Could you check a few things on this model? Use its own coordinates, in mm. A direction names the side the tool comes from. Coordinates: 2 decimals unless noted, no trailing zeros. Loops run counter-clockwise (first coordinate to the right, second up) from the corner with the lowest first, then second, coordinate; pieces in that order, holes last. Notation, with made-up numbers: M -16.5,-12 L 32.5,-12 A15 cw 32.5,13 Z; hole C 70.25,81 d6. An arc over 180 degrees is marked long. Return JSON: item names as keys, results as strings. Group by question number.
from build123d import *

# Parameters (mm, degrees)
SKETCH1_R                      = 27.4955
SKETCH1_R_2                    = 2
SKETCH1_R_3                    = 52.3875
SKETCH1_R_4                    = 3.3
BOSS_EXTRUDE1_DEPTH            = 9.525
M8_CLEARANCE_HOLE1_D           = 9
M8_CLEARANCE_HOLE1_CSINK_D     = 9.05
M8_CLEARANCE_HOLE1_CSINK_ANGLE = 90
CIRPATTERN1_COUNT              = 9


with BuildPart() as part:
    # Sketch1 → Boss-Extrude1 (new body)
    with BuildSketch(Plane(origin=(0, 0, 0), x_dir=(-1, 0, 0), z_dir=(0, 1, 0))):
        with BuildLine():
            Line((-663.918846707, 4.476573271), (-466.57213203, 18.457038772))
            ThreePointArc((-466.57213203, 18.457038772), (-462.140898161, 18.198594818), (-457.960546806, 16.706184206))
            ThreePointArc((-457.960546806, 16.706184206), (-450.250504554, 16.184701691), (-444.691176426, 21.552249203))
            Line((-444.691176426, 21.552249203), (-395.545795992, 142.743123059))
            ThreePointArc((-395.545795992, 142.743123059), (-394.045633102, 172.997422567), (-411.692336104, 197.617881552))
            ThreePointArc((-411.692336104, 197.617881552), (-413.372500119, 198.071242365), (-414.950136715, 197.336701751))
            Line((-414.950136715, 197.336701751), (-420.215020333, 192.071818133))
            ThreePointArc((-420.215020333, 192.071818133), (-427.298656721, 190.662795249), (-431.31121441, 196.668012211))
            Line((-431.31121441, 196.668012211), (-431.31121441, 203.240745001))
            ThreePointArc((-431.31121441, 203.240745001), (-431.968379704, 204.945600851), (-433.59982344, 205.768273949))
            ThreePointArc((-433.59982344, 205.768273949), (-438.15, 205.994), (-442.70017656, 205.768273949))
            ThreePointArc((-442.70017656, 205.768273949), (-444.331620296, 204.945600851), (-444.98878559, 203.240745001))
            Line((-444.98878559, 203.240745001), (-444.98878559, 196.668012211))
            ThreePointArc((-444.98878559, 196.668012211), (-451.48878559, 190.168012211), (-457.98878559, 196.668012211))
            Line((-457.98878559, 196.668012211), (-457.98878559, 197.245022653))
            ThreePointArc((-457.98878559, 197.245022653), (-459.278285753, 199.455870942), (-461.837486501, 199.421924563))
            ThreePointArc((-461.837486501, 199.421924563), (-464.019895008, 198.024699819), (-466.120112298, 196.506730383))
            Line((-466.120112298, 196.506730383), (-526.629683433, 150.121113421))
            ThreePointArc((-526.629683433, 150.121113421), (-551.530592574, 139.247052869), (-578.312485484, 134.661130809))
            ThreePointArc((-578.312485484, 134.661130809), (-599.244289514, 129.920579306), (-617.300018038, 118.318686532))
            ThreePointArc((-617.300018038, 118.318686532), (-626.772573796, 112.207783301), (-637.753125569, 109.658286556))
            Line((-637.753125569, 109.658286556), (-662.485690794, 106.73386739))
            ThreePointArc((-662.485690794, 106.73386739), (-670.168377129, 100.916938085), (-668.842832121, 91.372134981))
            Line((-668.842832121, 91.372134981), (-653.346537148, 71.746276485))
            ThreePointArc((-653.346537148, 71.746276485), (-651.347572908, 64.158994024), (-653.346537148, 56.571711562))
            Line((-653.346537148, 56.571711562), (-673.057822329, 18.34288652))
            ThreePointArc((-673.057822329, 18.34288652), (-672.544957076, 8.73610108), (-663.918846707, 4.476573271))
        make_face()
        with Locations(Location((-438.15, 160.02, 0), (0, 0, 270))):
            Circle(SKETCH1_R, mode=Mode.SUBTRACT)
        with Locations(Location((-632.402453753, 70.257452317, 0), (0, 0, 270))):
            Circle(SKETCH1_R_2, mode=Mode.SUBTRACT)
        with Locations(Location((-575.31, 72.821477372, 0), (0, 0, 270))):
            Circle(SKETCH1_R_3, mode=Mode.SUBTRACT)
        with Locations(Location((-661.367230642, 97.274762153, 0), (0, 0, 270))):
            Circle(SKETCH1_R_4, mode=Mode.SUBTRACT)
        with Locations(Location((-664.591931322, 13.977761728, 0), (0, 0, 270))):
            Circle(SKETCH1_R_4, mode=Mode.SUBTRACT)
        with Locations(Location((-453.518014272, 25.131712658, 0), (0, 0, 270))):
            Circle(SKETCH1_R_4, mode=Mode.SUBTRACT)
        with BuildLine():
            ThreePointArc((-518.217546247, 72.257452317), (-520.217546247, 70.257452317), (-518.217546247, 68.257452317))
            ThreePointArc((-518.217546247, 68.257452317), (-516.217546247, 70.257452317), (-518.217546247, 72.257452317))
        make_face(mode=Mode.SUBTRACT)
        with BuildLine():
            ThreePointArc((-575.31, 17.671477372), (-577.31, 15.671477372), (-575.31, 13.671477372))
            ThreePointArc((-575.31, 13.671477372), (-573.31, 15.671477372), (-575.31, 17.671477372))
        make_face(mode=Mode.SUBTRACT)
        with BuildLine():
            ThreePointArc((-575.31, 131.971477372), (-577.31, 129.971477372), (-575.31, 127.971477372))
            ThreePointArc((-575.31, 127.971477372), (-573.31, 129.971477372), (-575.31, 131.971477372))
        make_face(mode=Mode.SUBTRACT)
    extrude(amount=BOSS_EXTRUDE1_DEPTH)

    # M8 Clearance Hole1 (through all)
    with Locations(Plane(origin=(0, 0, 0), x_dir=(-1, 0, 0), z_dir=(0, -1, 0))):
        with Locations((-438.15, -199.019999978)):
            m8_clearance_hole1 = CounterSinkHole(M8_CLEARANCE_HOLE1_D / 2, M8_CLEARANCE_HOLE1_CSINK_D / 2, counter_sink_angle=M8_CLEARANCE_HOLE1_CSINK_ANGLE)

    # CirPattern1: M8 Clearance Hole1 ×9 about axis
    cirpattern1_axis = Axis((438.15, 0, 160.02), (0, 1, 0))
    for i in range(1, CIRPATTERN1_COUNT):
        add(m8_clearance_hole1.rotate(cirpattern1_axis, i * 360 / CIRPATTERN1_COUNT), mode=Mode.SUBTRACT)


solid = part.part
(1) For faces 1 (the face through (566.63, 4.7, 11.37)), 2 (the face through (598.965, 4.696, 130.037)), which set-ups out of +Z, -Z, +X, -X, +Y, -Y let a thin tool reach every point of the face, with its end or its side?
(2) We'd pull the mould along Z, two halves only. Please class faces 3 (the face through (450.355, 4.696, 16.147)), 4 (the face through (672.62, 4.7, 8.85)), 5 (the face through (450.246, 4.696, 25.561)): +Z half, -Z half, draft (parallel to the pull), parting line (faces both ways), or undercut.
(3) If I drill on L1, parallel to Z at x = 455.5, y = 3; L2, parallel to Z at x = 576, y = 2; L3, parallel to X at y = 3.5, z = 163, over which ranges is the centre line in solid material (lowest first)? Write a range as [from, to].
(4) Will these pins go through, and if not, where does the flat tip stop? P1, Ø8, axis at x = 404.38, z = 140.52, coming from the -Y side; P2, Ø6.5, axis at x = 575.31, z = 129.97, coming from the -Y side; P3, Ø4, axis at x = 480.5, y = 2, coming from the +Z side; P4, Ø0.6, axis at y = 5.5, z = 197, coming from the -X side.
(5) Imagine slicing it at B-B, the plane z = 80. Write out the boundary of the cut face in (x, y) (3 decimals), then the cut area to 3 significant figures.
(6) Imagine slicing it at C-C, the plane x = 438.15. Count the separate pieces of the cut face and the enclosed holes in it, then the cut area to 3 significant figures.
(7) Imagine slicing it at A-A, the plane x = 588.5. Write out the boundary of the cut face in (y, z) (3 decimals).
Checks:
{
 "1": {"face 1": "-Z, +Y, -Y", "face 2": "+Z, +X, +Y, -Y"},
 "2": {"face 3": "-Z half", "face 4": "parting line", "face 5": "undercut"},
 "3": {"L1": "[15.82, 22.49], [27.77, 121.33], [125.41, 138.69], [181.35, 191.55]", "L2": "[10.7, 13.79], [17.55, 20.44], [125.2, 128.09], [131.85, 134.8]", "L3": "[392.27, 397.32], [402.17, 410.82], [465.48, 474.13], [478.98, 509.83]"},
 "4": {"P1": "through", "P2": "y = 0", "P3": "z = 187.02", "P4": "x = 410.43"},
 "5": {"outline": "M 420.989,0 L 523.417,0 L 523.417,9.525 L 420.989,9.525 Z; M 627.203,0 L 659.864,0 L 659.864,9.525 L 627.203,9.525 Z", "area": "1,290 mm²"},
 "6": {"separate pieces": "3", "enclosed holes": "0", "area": "994 mm²"},
 "7": {"outline": "M 0,9.819 L 9.525,9.819 L 9.525,22.122 L 0,22.122 Z; M 0,123.521 L 9.525,123.521 L 9.525,133.313 L 0,133.313 Z"}
}
